Build history of the part. All positions in model axes, mm. A direction names the side the tool comes from. Round coordinates to 2 decimals unless told otherwise and drop trailing zeros. Loops run counter-clockwise (first coordinate to the right, second up) from the corner with the lowest first, then second, coordinate; pieces in that order, holes last. Notation, with made-up numbers: (-40, 35.25) - (-9, 35.25) arc R21 cw to (-9, 67.25) - close; hole circle Ø7 at (74.5, 1.25). An arc over 180 degrees is marked (long way). Put each result on its own line as item: value. Start each with the question number.
from build123d import *

# Parameters (mm, degrees)
SKETCH1_R           = 7.5
SKETCH1_R_2         = 4
BOSS_EXTRUDE1_DEPTH = 10
SKETCH3_R           = 12.5
SKETCH3_R_2         = 4
BOSS_EXTRUDE2_DEPTH = 5
SKETCH4_R           = 7.5
SKETCH4_R_2         = 4
BOSS_EXTRUDE3_DEPTH = 10
SKETCH5_R           = 1
CUT_EXTRUDE1_DEPTH  = 10


with BuildPart() as part:
    # Sketch1 → Boss-Extrude1 (new body)
    with BuildSketch(Plane.XY):
        Circle(SKETCH1_R)
        Circle(SKETCH1_R_2, mode=Mode.SUBTRACT)
    extrude(amount=BOSS_EXTRUDE1_DEPTH)

    # Sketch3 → Boss-Extrude2 (add)
    with BuildSketch(Plane.XY.offset(10)):
        Circle(SKETCH3_R)
        Circle(SKETCH3_R_2, mode=Mode.SUBTRACT)
    extrude(amount=BOSS_EXTRUDE2_DEPTH)

    # Sketch4 → Boss-Extrude3 (add)
    with BuildSketch(Plane.XY.offset(15)):
        Circle(SKETCH4_R)
        Circle(SKETCH4_R_2, mode=Mode.SUBTRACT)
    extrude(amount=BOSS_EXTRUDE3_DEPTH)

    # Sketch5 → Cut-Extrude1 (cut)
    with BuildSketch(Plane(origin=(0, 0, 0), x_dir=(0, 0, -1), z_dir=(1, 0, 0))):
        with Locations(Location((-20, 0, 0), (0, 0, 180))):
            Circle(SKETCH5_R)
    extrude(amount=-CUT_EXTRUDE1_DEPTH, mode=Mode.SUBTRACT)


solid = part.part
1) Slice it at B-B, the plane x = 0. Write the cut outline in (y, z).
2) Drill centre lines: line 1 (Y direction, x = 0, z = 14.25); line 2 (X direction, y = 0.25, z = 5.5); line 3 (Z direction, x = -8.75, y = -1.25). Where is each one in solid material? Low to high. Write a range as [from, to].
3) Slice it at A-A, the plane y = 0. Write the cut outline in (x, z), and give its area (3 significant figures).
4) Slice it at D-D, the plane z = 6.5. Write the cut outline in (x, y).
5) Which spindle directions (+Z, -Z, +X, -X, +Y, -Y) get a long thin tool onto all of the face, cutting with end or side? Do faces 1 (the face through (-6, 0, 19)), 2 (the face through (0, -8, 10)), 3 (the face through (3, -3, 0)), 4 (the face through (0, -8, 15)). Say none if no direction does.
6) Drop flat-ended pins along their axis: pin 1 Ø2 at (y, z) = (-4.5, 19.5) entering from -X; pin 2 Ø8 at (y, z) = (6.5, 22) entering from +X; pin 3 Ø2 at (y, z) = (-4.5, 8) entering from +X; pin 4 Ø7.5 at (x, y) = (-1, -2.5) entering from -Z. Give the stop position or say it passes through.
7) Pull direction Y, two halves, no side cores. Call faces 5 (the face through (3, -3, 25)), 6 (the face through (3.695, -1.532, 12.325)), 7 (the face through (11.923, 3.755, 12.465)): pulls with the +Y half, pulls with the -Y half, needs draft (parallel to the pull), parting line crosses it, or undercut.
8) Slice it at C-C, the plane x = -7. Write the cut outline in (y, z).
Taken from the geometry:
1. outline: (-12.5, 10) - (-7.5, 10) - (-7.5, 0) - (-4, 0) - (-4, 25) - (-7.5, 25) - (-7.5, 15) - (-12.5, 15) - close; (4, 0) - (7.5, 0) - (7.5, 10) - (12.5, 10) - (12.5, 15) - (7.5, 15) - (7.5, 25) - (4, 25) - close
2. line 1: y = [-12.5, -4], [4, 12.5]
2. line 2: x = [-7.5, -3.99], [3.99, 7.5]
2. line 3: z = [10, 15]
3. outline: (-12.5, 10) - (-7.5, 10) - (-7.5, 0) - (-4, 0) - (-4, 19) - (-7.5, 19) - (-7.5, 15) - (-12.5, 15) - close; (-7.5, 21) - (-4, 21) - (-4, 25) - (-7.5, 25) - close; (4, 0) - (7.5, 0) - (7.5, 10) - (12.5, 10) - (12.5, 15) - (7.5, 15) - (7.5, 25) - (4, 25) - close
3. area: 218 mm2
4. outline: circle Ø15 at (0, 0); hole circle Ø8 at (0, 0)
5. face 1: -X
5. face 2: -Z
5. face 3: -Z, +X, -X, +Y, -Y
5. face 4: +Z
6. pin 1: stops at x = -6.63
6. pin 2: stops at x = 7.07
6. pin 3: stops at x = 6.63
6. pin 4: stops at z = 0
7. face 5: needs draft
7. face 6: undercut
7. face 7: parting line crosses it
8. outline: (-10.36, 10) - (-2.69, 10) - (-2.69, 0) - (2.69, 0) - (2.69, 10) - (10.36, 10) - (10.36, 15) - (2.69, 15) - (2.69, 25) - (-2.69, 25) - (-2.69, 15) - (-10.36, 15) - close; hole circle Ø2 at (0, 20)
